Could you check a few things on this model? Use its own coordinates, in mm. A direction names the side the tool comes from. Coordinates: 2 decimals unless noted, no trailing zeros. Loops run counter-clockwise (first coordinate to the right, second up) from the corner with the lowest first, then second, coordinate; pieces in that order, holes last. Notation, with made-up numbers: M -27,-7.5 L 6,-7.5 A21 cw 6,31.5 Z; hole C 13,62 d3. An arc over 180 degrees is marked long. Write each question's results on one line, items separated by ' | '.
```python
from build123d import *

# Parameters (mm, degrees)
SKETCH2_R           = 50
SKETCH2_R_2         = 15
BOSS_EXTRUDE1_DEPTH = 200
BOSS_EXTRUDE2_DEPTH = 40
SKETCH4_W           = 40
SKETCH4_H           = 100
BOSS_EXTRUDE3_DEPTH = 120
CHAMFER1_SIZE       = 50
CHAMFER2_SIZE       = 50


with BuildPart() as part:
    # Sketch2 → Boss-Extrude1 (new body)
    with BuildSketch(Plane.XY):
        Circle(SKETCH2_R)
        Circle(SKETCH2_R_2, mode=Mode.SUBTRACT)
    extrude(amount=BOSS_EXTRUDE1_DEPTH)

    # Sketch3 → Boss-Extrude2 (add)
    with BuildSketch(Plane(origin=(0, 0, 0), x_dir=(-1, 0, 0), z_dir=(0, 0, -1))):
        Polygon((-150, 50), (-150, 33.43588559), (-150, -50), (150, -50), (150, 50), align=None)
    extrude(amount=BOSS_EXTRUDE2_DEPTH)

    # Sketch4 → Boss-Extrude3 (add)
    with BuildSketch(Plane(origin=(0, 0, -40), x_dir=(-1, 0, 0), z_dir=(0, 0, -1))):
        Polygon((110, 50), (110, 33.823115264), (110, -50), (150, -50), (150, 50), align=None)
        with Locations((-130, 0)):
            Rectangle(SKETCH4_W, SKETCH4_H)
    extrude(amount=BOSS_EXTRUDE3_DEPTH)

    # Chamfer1
    # the kernel refuses this chamfer: 50 mm, written as the material it takes off along each edge
    with BuildSketch(Plane(origin=(-150, -178.584149398, -160), x_dir=(0.9996219169112966, 0, -0.027495876610586594), z_dir=(0, 1, 0))) as chamfer1_piece_1:
        Polygon((CHAMFER1_SIZE * 0.999621916911, -CHAMFER1_SIZE * 0.0274958766106), (-CHAMFER1_SIZE * 0.0274958766106, -CHAMFER1_SIZE * 0.999621916911), (0, 0), align=None)
    extrude(amount=357.168298797, mode=Mode.SUBTRACT)

    # Chamfer2
    # the kernel refuses this chamfer: 50 mm, written as the material it takes off along each edge
    with BuildSketch(Plane(origin=(150, -178.584149398, -160), x_dir=(0.027495876610586594, 0, 0.9996219169112966), z_dir=(0, 1, 0))) as chamfer2_piece_1:
        Polygon((CHAMFER2_SIZE * 0.999621916911, -CHAMFER2_SIZE * 0.0274958766106), (-CHAMFER2_SIZE * 0.0274958766106, -CHAMFER2_SIZE * 0.999621916911), (0, 0), align=None)
    extrude(amount=357.168298797, mode=Mode.SUBTRACT)


solid = part.part
```
(1) Which directions (+Z, -Z, +X, -X, +Y, -Y) give clear straight access to the entire face, cutting with the end or side of a thin tool? Please do faces 1 (the flat face through (2, 1, -40)), 2 (the flat face through (0, 0, 0)), 3 (the flat face through (2, -50, -24)).
Reported:
face 1: -Z, +Y, -Y | face 2: +Z | face 3: +Z, -Z, +X, -X, -Y
(2) Imagine slicing it at D-D, the plane x = -21. List the corners of the cut face in (y, z) for me, and give its area (3 significant figures).
Reported:
outline: M -50,-40 L 50,-40 L 50,0 L 45.38,0 L 45.38,200 L -45.38,200 L -45.38,0 L -50,0 Z | area: 22,200 mm2
(3) Imagine slicing it at B-B, the plane y = 42. List the corners of the cut face in (x, z) for me, and give its area (3 significant figures).
Reported:
outline: M -150,-110 L -110,-150 L -110,-40 L 110,-40 L 110,-150 L 150,-110 L 150,0 L 27.13,0 L 27.13,200 L -27.13,200 L -27.13,0 L -150,0 Z | area: 30,100 mm2
(4) Will these pins go through, and if not, where does the flat tip stop? P1, Ø2, axis at x = -11.5, z = 128.5, coming from the +Y side; P2, Ø1.5, axis at x = -42, z = 137.5, coming from the +Y side; P3, Ø8, axis at x = -25, z = 5, coming from the -Y side.
Reported:
P1: stops at y = 48.89 | P2: stops at y = 28.26 | P3: stops at y = -45.38
(5) Imagine slicing it at C-C, the plane z = 79.5. List the corners of the cut face in (x, y) for me, and give its area (3 significant figures).
Reported:
outline: C 0,0 d100; hole C 0,0 d30 | area: 7,150 mm2
(6) Imagine slicing it at A-A, the plane z = -84. List the corners of the cut face in (x, y) for me.
Reported:
outline: M -150,-50 L -110,-50 L -110,50 L -150,50 Z; M 110,-50 L 150,-50 L 150,50 L 110,50 Z
(7) Please list where these lines run through material, in increasing order: probe 1 along Y at (x, z) = (0, 62); probe 2 along X at (y, z) = (-9.5, 125); probe 3 along Z at (x, y) = (84, 32). Write a range as from..to.
Reported:
probe 1: y = -50..-15, 15..50 | probe 2: x = -49.09..-11.61, 11.61..49.09 | probe 3: z = -40..0
(8) If we mould it in two halves opening along X, with no side actions, what happens to faces 4 (the flat face through (-150, -1, -54)), 5 (the flat face through (-12, -10, 200)), 6 (the cylindrical face through (-14.985, 0.66, 98.6)), 7 (the flat face through (130, -1, -130))? For each: released by +X, released by -X, zero draft, split by the parting line, or undercut.
Reported:
face 4: released by -X | face 5: zero draft | face 6: undercut | face 7: released by +X
